```python
from build123d import *

# Parameters (mm, degrees)
SKETCH1_W           = 6.95
SKETCH1_H           = 6.75
BOSS_EXTRUDE1_DEPTH = 4.6
SKETCH3_3_R         = 2.685665185
CUT_EXTRUDE3_DEPTH  = 0.05
SKETCH3_4_R         = 2.471595258
CUT_EXTRUDE4_DEPTH  = 1
SKETCH3_R           = 0.249549506
CUT_EXTRUDE5_DEPTH  = 0.5


with BuildPart() as part:
    # Sketch1 → Boss-Extrude1 (new body)
    with BuildSketch(Plane(origin=(0, 0, 0), x_dir=(1, 0, 0), z_dir=(0, 1, 0))):
        with Locations((-3.475, 3.375)):
            Rectangle(SKETCH1_W, SKETCH1_H)
    extrude(amount=BOSS_EXTRUDE1_DEPTH)

    # Sketch3<3> → Cut-Extrude3 (cut)
    with BuildSketch(Plane(origin=(0, 4.6, 0), x_dir=(1, 0, 0), z_dir=(0, 1, 0))):
        with BuildLine():
            Line((-2.404106083, 6.015623034), (-2.312667033, 6.241094539))
            Line((-2.312667033, 6.241094539), (-2.227566093, 6.2065822))
            Line((-2.227566093, 6.2065822), (-2.326206207, 5.982676477))
            ThreePointArc((-2.326206207, 5.982676477), (-1.890758445, 5.743519048), (-1.50346617, 5.432366798))
            Line((-1.50346617, 5.432366798), (-1.330630635, 5.60014662))
            Line((-1.330630635, 5.60014662), (-1.258910519, 5.52626536))
            Line((-1.258910519, 5.52626536), (-1.430410767, 5.359781765))
            ThreePointArc((-1.430410767, 5.359781765), (-1.122158532, 4.982432988), (-0.882700889, 4.558084573))
            Line((-0.882700889, 4.558084573), (-0.665701499, 4.657119684))
            Line((-0.665701499, 4.657119684), (-0.615961925, 4.534471247))
            Line((-0.615961925, 4.534471247), (-0.834376966, 4.445893916))
            ThreePointArc((-0.834376966, 4.445893916), (-0.689137564, 3.973894209), (-0.627572536, 3.483906499))
            Line((-0.627572536, 3.483906499), (-0.302033066, 3.483906499))
            Line((-0.302033066, 3.483906499), (-0.302033066, 3.301563496))
            Line((-0.302033066, 3.301563496), (-0.626437053, 3.301563496))
            ThreePointArc((-0.626437053, 3.301563496), (-0.685462224, 2.793465152), (-0.834376966, 2.304106084))
            Line((-0.834376966, 2.304106084), (-0.615961925, 2.215528753))
            Line((-0.615961925, 2.215528753), (-0.665701499, 2.092880316))
            Line((-0.665701499, 2.092880316), (-0.882700889, 2.191915427))
            ThreePointArc((-0.882700889, 2.191915427), (-1.122158532, 1.767567012), (-1.430410767, 1.390218235))
            Line((-1.430410767, 1.390218235), (-1.258910519, 1.22373464))
            Line((-1.258910519, 1.22373464), (-1.330630635, 1.14985338))
            Line((-1.330630635, 1.14985338), (-1.50346617, 1.317633202))
            ThreePointArc((-1.50346617, 1.317633202), (-3.475, 0.525490606), (-5.44653383, 1.317633202))
            Line((-5.44653383, 1.317633202), (-5.619369365, 1.14985338))
            Line((-5.619369365, 1.14985338), (-5.691089481, 1.22373464))
            Line((-5.691089481, 1.22373464), (-5.519589233, 1.390218235))
            ThreePointArc((-5.519589233, 1.390218235), (-5.827841468, 1.767567012), (-6.067299111, 2.191915427))
            Line((-6.067299111, 2.191915427), (-6.284298501, 2.092880316))
            Line((-6.284298501, 2.092880316), (-6.334038075, 2.215528753))
            Line((-6.334038075, 2.215528753), (-6.115623034, 2.304106084))
            ThreePointArc((-6.115623034, 2.304106084), (-6.264537776, 2.793465152), (-6.323562947, 3.301563496))
            Line((-6.323562947, 3.301563496), (-6.647966934, 3.301563496))
            Line((-6.647966934, 3.301563496), (-6.647966934, 3.483906499))
            Line((-6.647966934, 3.483906499), (-6.322427464, 3.483906499))
            ThreePointArc((-6.322427464, 3.483906499), (-6.260862436, 3.973894209), (-6.115623034, 4.445893916))
            Line((-6.115623034, 4.445893916), (-6.334038075, 4.534471247))
            Line((-6.334038075, 4.534471247), (-6.284298501, 4.657119684))
            Line((-6.284298501, 4.657119684), (-6.067299111, 4.558084573))
            ThreePointArc((-6.067299111, 4.558084573), (-5.827841468, 4.982432988), (-5.519589233, 5.359781765))
            Line((-5.519589233, 5.359781765), (-5.691089481, 5.52626536))
            Line((-5.691089481, 5.52626536), (-5.619369365, 5.60014662))
            Line((-5.619369365, 5.60014662), (-5.44653383, 5.432366798))
            ThreePointArc((-5.44653383, 5.432366798), (-5.059241555, 5.743519048), (-4.623793793, 5.982676477))
            Line((-4.623793793, 5.982676477), (-4.722433907, 6.2065822))
            Line((-4.722433907, 6.2065822), (-4.637332967, 6.241094539))
            Line((-4.637332967, 6.241094539), (-4.545893917, 6.015623034))
            ThreePointArc((-4.545893917, 6.015623034), (-4.079985397, 6.159546005), (-3.596359951, 6.221923875))
            Line((-3.596359951, 6.221923875), (-3.596359951, 6.550048868))
            Line((-3.596359951, 6.550048868), (-3.475, 6.550048868))
            Line((-3.475, 6.550048868), (-3.475, 6.224509394))
            ThreePointArc((-3.475, 6.224509394), (-2.929461896, 6.171800308), (-2.404106083, 6.015623034))
        make_face()
        with Locations((-3.475, 3.375)):
            Circle(SKETCH3_3_R, mode=Mode.SUBTRACT)
    extrude(amount=-CUT_EXTRUDE3_DEPTH, mode=Mode.SUBTRACT)

    # Sketch3<4> → Cut-Extrude4 (cut)
    with BuildSketch(Plane(origin=(0, 4.6, 0), x_dir=(1, 0, 0), z_dir=(0, 1, 0))):
        with Locations((-3.475, 3.375)):
            Circle(SKETCH3_4_R)
    extrude(amount=-CUT_EXTRUDE4_DEPTH, mode=Mode.SUBTRACT)

    # Sketch3 → Cut-Extrude5 (cut)
    with BuildSketch(Plane(origin=(0, 4.6, 0), x_dir=(1, 0, 0), z_dir=(0, 1, 0))):
        with Locations((-0.615961925, 6.280685908)):
            Circle(SKETCH3_R)
    extrude(amount=-CUT_EXTRUDE5_DEPTH, mode=Mode.SUBTRACT)


solid = part.part
```
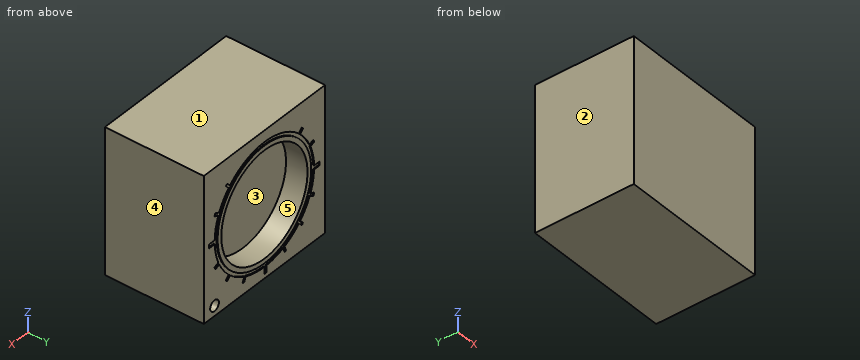
Geometry: final body of the model. Coordinates: model frame, mm. Face numbers are marked on the shaded views. A direction names the side the tool comes from. Round coordinates to 2 decimals unless told otherwise and drop trailing zeros. Order: outer loops, then holes, each group sorted by start corner. A loop starts at its lowest first (then second) coordinate and runs counter-clockwise, first axis right, second up. Notation, with made-up numbers: (86, 22.25) -> (118, 22.25) arc R25 cw to (118, 41.25) -> close; hole circle Ø3 at (7.25, -18). An arc over 180 degrees is marked (long way). Write each question's results on one line, items separated by ' | '.
Q1. Section query B-B (x = -5.25). Output: boundary loops of the cut face in (y, z), and give its area (3 significant figures).
Response values:
outline: (0, -6.75) -> (4.6, -6.75) -> (4.6, -5.6) -> (4.55, -5.6) -> (4.55, -5.39) -> (4.6, -5.39) -> (4.6, -5.09) -> (3.6, -5.09) -> (3.6, -1.66) -> (4.6, -1.66) -> (4.6, -1.36) -> (4.55, -1.36) -> (4.55, -1.15) -> (4.6, -1.15) -> (4.6, 0) -> (0, 0) -> close | area: 27.6 mm²
Q2. Pull-direction query (X, two-part tool) for the marked faces 1, 2 and 3; classes: released by +X, released by -X, zero draft, split by the parting line, or undercut.
Response values:
face 1: zero draft | face 2: released by -X | face 3: undercut
Q3. Ray query, line 1 along Y through (x, z) = (-3.75, -1.25); line 2 along X through (y, z) = (4.2, -4.5); line 3 along Z through (x, y) = (-4, 3.8). Return the intervals inside material, ascending.
Response values:
line 1: 0 to 3.6 | line 2: -6.95 to -5.68, -1.27 to 0 | line 3: -6.75 to -5.79, -0.96 to 0
Q4. Section query A-A (z = -5.75). Output: boundary loops of the cut face in (x, y), and give its area (3 significant figures).
Response values:
outline: (-6.95, 0) -> (0, 0) -> (0, 4.6) -> (-1.9, 4.6) -> (-1.9, 4.55) -> (-2.22, 4.55) -> (-2.22, 4.6) -> (-2.79, 4.6) -> (-2.79, 3.6) -> (-4.16, 3.6) -> (-4.16, 4.6) -> (-4.73, 4.6) -> (-4.73, 4.55) -> (-5.05, 4.55) -> (-5.05, 4.6) -> (-6.95, 4.6) -> close | area: 30.6 mm²
Q5. Access query for the marked faces 4 and 5. Directions: +Z, -Z, +X, -X, +Y, -Y. A direction counts if a zero-diameter tool reaches every point of the face in a straight line with its end or side. Return the directions, or none.
Response values:
face 4: +Z, -Z, +X, +Y, -Y | face 5: +Y
Q6. Section query C-C (y = 3.95). Output: boundary loops of the cut face in (x, z) (3 decimals).
Response values:
outline: (-6.95, -6.75) -> (0, -6.75) -> (0, 0) -> (-6.95, 0) -> close; hole circle Ø4.943 at (-3.475, -3.375)
